Verification items for the finished model (mm, model axes). Round coordinates to 2 decimals unless told otherwise and drop trailing zeros. Write each loop counter-clockwise with the first axis right and the second up, starting at its lowest first coordinate (ties: lowest second). Pieces come first, ordered by that corner, then holes. Notation, with made-up numbers: M -8,55.25 L 12,55.25 A5 ccw 12,61.25 Z; hole C 3.5,22 d9. An arc over 180 degrees is marked long. One line per item, written item: value. Start each with the question number.
Item 1: Section check B-B, the plane y = 0.35. Record the cut outline in (x, z), then the cut area to 3 significant figures.
Item 2: Thickness scan on probe 1 along X at (y, z) = (0.45, -40.15); probe 2 along Z at (x, y) = (-50, 1). Record the ranges inside material, lowest first. Write a range as from..to.
Item 3: Section check A-A, the plane z = -40.2. Record the cut outline in (x, y).
from build123d import *

# Parameters (mm, degrees)
SKETCH1_R           = 0.4
BOSS_EXTRUDE1_DEPTH = 1.5


with BuildPart() as part:
    # Sketch1 → Boss-Extrude1 (new body)
    with BuildSketch(Plane(origin=(0, 0, 0), x_dir=(1, 0, 0), z_dir=(0, 1, 0))):
        Polygon((-55.29426973, 39.238190042), (-40.301565833, 39.238190042), (-40.301565833, 40.850641592), (-55.29426973, 40.850641592), (-55.29426973, 40.044415817), align=None)
        with BuildLine():
            ThreePointArc((-51.901565833, 40.044415817), (-52.301565833, 39.644415817), (-52.701565833, 40.044415817))
            ThreePointArc((-52.701565833, 40.044415817), (-52.301565833, 40.444415817), (-51.901565833, 40.044415817))
        make_face(mode=Mode.SUBTRACT)
        with Locations(Location((-45.301565833, 40.044415817, 0), (0, 0, 270))):
            Circle(SKETCH1_R, mode=Mode.SUBTRACT)
        with BuildLine():
            ThreePointArc((-53.901565833, 40.044415817), (-54.301565833, 39.644415817), (-54.701565833, 40.044415817))
            ThreePointArc((-54.701565833, 40.044415817), (-54.301565833, 40.444415817), (-53.901565833, 40.044415817))
        make_face(mode=Mode.SUBTRACT)
        with Locations(Location((-50.301565833, 40.044415817, 0), (0, 0, 270))):
            Circle(SKETCH1_R, mode=Mode.SUBTRACT)
        with Locations(Location((-42.801565833, 40.044415817, 0), (0, 0, 270))):
            Circle(SKETCH1_R, mode=Mode.SUBTRACT)
    extrude(amount=BOSS_EXTRUDE1_DEPTH)


solid = part.part
Response values:
1. outline: M -55.29,-40.85 L -40.3,-40.85 L -40.3,-39.24 L -55.29,-39.24 Z; hole C -54.3,-40.04 d0.8; hole C -52.3,-40.04 d0.8; hole C -50.3,-40.04 d0.8; hole C -45.3,-40.04 d0.8; hole C -42.8,-40.04 d0.8
1. area: 21.7 mm2
2. probe 1: x = -55.29..-54.69, -53.92..-52.69, -51.92..-50.69, -49.92..-45.69, -44.92..-43.19, -42.42..-40.3
2. probe 2: z = -40.85..-40.31, -39.78..-39.24
3. outline: M -55.29,0 L -54.67,0 L -54.67,1.5 L -55.29,1.5 Z; M -53.93,0 L -52.67,0 L -52.67,1.5 L -53.93,1.5 Z; M -51.93,0 L -50.67,0 L -50.67,1.5 L -51.93,1.5 Z; M -49.93,0 L -45.67,0 L -45.67,1.5 L -49.93,1.5 Z; M -44.93,0 L -43.17,0 L -43.17,1.5 L -44.93,1.5 Z; M -42.43,0 L -40.3,0 L -40.3,1.5 L -42.43,1.5 Z
